Part model, mm, in its own coordinate system. Face numbers are marked on the shaded views. Give positions to 0.01 mm unless a question says otherwise; leave off trailing zeros. Order: outer loops, then holes, each group sorted by start corner. A loop starts at its lowest first (then second) coordinate and runs counter-clockwise, first axis right, second up. Notation, with made-up numbers: (-39, -30) - (-30, -30) arc R25 ccw to (-30, -8) - close; hole circle Ø6 at (80.5, 53). An arc over 180 degrees is marked (long way). One line per item, written item: value.
Autodesk Inventor part; units mm, degrees
ref_plane "YZ Plane" through (0, 0, 0) normal (1, 0, 0) x (0, 1, 0)
ref_plane "XZ Plane" through (0, 0, 0) normal (0, 1, 0) x (-1, 0, 0)
ref_plane "XY Plane" through (0, 0, 0) normal (0, 0, 1) x (1, 0, 0)
sketch "Sketch1" plane through (0, 0, 0) normal (0, 0, 1) x (1, 0, 0)
  line L0 (0, 0) -> (38, 0)
  line L1 (38, 0) -> (38, 37)
  line L2 (38, 37) -> (0, 37)
  line L3 (0, 37) -> (0, 0)
  line L4 (19, 37) -> (19, 0) construction
  circle A0 centre (11, 4) radius 2.5
  circle A1 centre (27, 4) radius 2.5
  circle A2 centre (19, 8) radius 2
  circle A3 centre (19, 16) radius 2
  circle A4 centre (19, 24) radius 3.5
  circle A5 centre (19, 33) radius 2
  circle A6 centre (3, 24) radius 2
  circle A7 centre (35, 24) radius 2
  dimension "d0" = 38
  dimension "d1" = 37
  dimension "d2" = 5
  dimension "d3" = 8
  dimension "d4" = 4
  dimension "d5" = 5
  dimension "d6" = 8
  dimension "d7" = 4
  dimension "d8" = 4
  dimension "d9" = 8
  dimension "d10" = 4
  dimension "d11" = 16
  dimension "d12" = 7
  dimension "d13" = 24
  dimension "d14" = 4
  dimension "d15" = 17
  dimension "d18" = 4
  dimension "d19" = 4
  dimension "d20" = 32
  dimension "d21" = 3
  dimension "d22" = 13
  dimension "d23" = 13
extrude "Extrusion1" add sketch "Sketch1" along normal blind 3
thread "Thread1"
thread "Thread2"
thread "Thread3"
thread "Thread4"
thread "Thread5"
fillet "Fillet1" radius 1 2 edges at (17, 33, 3) (17, 16, 3)
properties part number "DC Motor-25 Bracket B-Blue" material "Aluminum 6061"
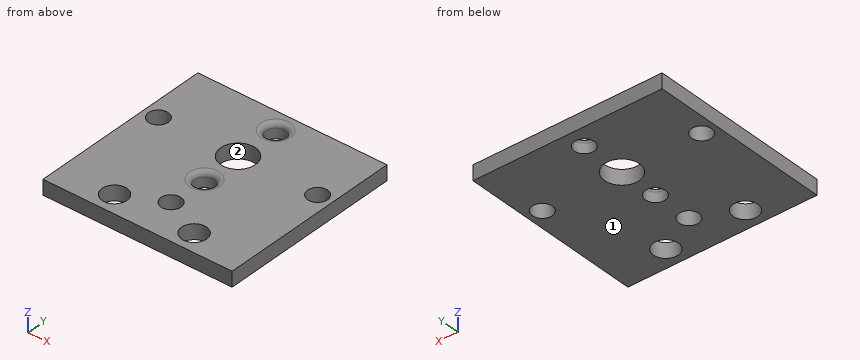
1) Drill centre lines: line 1 along Y through (x, z) = (19, 1.55); line 2 along Y through (x, z) = (11, 1.3); line 3 along Y through (x, z) = (20.5, 2.25). Where is each one in solid material? Low to high. Write a range as from..to.
Outcome:
line 1: y = 0..6, 10..14, 18..20.5, 27.5..31, 35..37
line 2: y = 0..1.5, 6.5..37
line 3: y = 0..6.68, 9.32..14.63, 17.37..20.84, 27.16..31.63, 34.37..37
2) Cut at D-D, the plane x = 35. Give the cut face in (y, z).
Outcome:
outline: (0, 0) - (22, 0) - (22, 3) - (0, 3) - close; (26, 0) - (37, 0) - (37, 3) - (26, 3) - close
3) Pin check, flat tip, straight feed: pin 1 (4.5 mm diameter, centred on x = 11, y = 4, fed in from -Z). Stop position of the tip, or through.
Outcome:
pin 1: passes through
4) Cut at A-A, the plane x = 27. Give the cut face in (y, z), then the cut area to 3 significant figures.
Outcome:
outline: (0, 0) - (1.5, 0) - (1.5, 3) - (0, 3) - close; (6.5, 0) - (37, 0) - (37, 3) - (6.5, 3) - close
area: 96.0 mm^2
5) Cut at B-B, the plane y = 33. Give the cut face in (x, z).
Outcome:
outline: (0, 0) - (17, 0) - (17, 2) arc R1 ccw to (16, 3) - (0, 3) - close; (21, 0) - (38, 0) - (38, 3) - (22, 3) arc R1 ccw to (21, 2) - close
6) Cut at C-C, the plane x = 19. Give the cut face in (y, z), then the cut area to 3 significant figures.
Outcome:
outline: (0, 0) - (6, 0) - (6, 3) - (0, 3) - close; (10, 0) - (14, 0) - (14, 2) arc R1 ccw to (13, 3) - (10, 3) - close; (18, 0) - (20.5, 0) - (20.5, 3) - (19, 3) arc R1 ccw to (18, 2) - close; (27.5, 0) - (31, 0) - (31, 2) arc R1 ccw to (30, 3) - (27.5, 3) - close; (35, 0) - (37, 0) - (37, 3) - (36, 3) arc R1 ccw to (35, 2) - close
area: 53.1 mm^2
7) Mould opens along Y. For the marked faces 1 and 2 say: released by +Y, released by -Y, zero draft, split by the parting line, or undercut.
Outcome:
face 1: zero draft
face 2: undercut
